```python
from build123d import *

# Parameters (mm, degrees)
SKETCH2_W               = 101.6
SKETCH2_H               = 25.4
BOSS_EXTRUDE1_DEPTH     = 6.35
SKETCH3_R               = 6.35
CUT_EXTRUDE1_DEPTH      = 3.81
CUT_EXTRUDE2_DEPTH      = 53.74706153
CUT_EXTRUDE2_DEPTH_BACK = 6.35
CUT_EXTRUDE3_DEPTH      = 53.74706153
CUT_EXTRUDE3_DEPTH_BACK = 6.35


with BuildPart() as part:
    # Sketch2 → Boss-Extrude1 (new body)
    with BuildSketch(Plane(origin=(0, 0, 0), x_dir=(1, 0, 0), z_dir=(0, 1, 0))):
        Rectangle(SKETCH2_W, SKETCH2_H)
    extrude(amount=BOSS_EXTRUDE1_DEPTH)

    # Sketch3 → Cut-Extrude1 (cut)
    with BuildSketch(Plane.XZ):
        with Locations(Location((-38.1, 0, 0), (0, 0, 270))):
            Circle(SKETCH3_R)
    extrude(amount=-CUT_EXTRUDE1_DEPTH, mode=Mode.SUBTRACT)

    # Sketch4 → Cut-Extrude2 (cut, two sides: drawn at the far end of the back side and taken through both)
    with BuildSketch(Plane(origin=(0, 6.35, 0), x_dir=(1, 0, 0), z_dir=(0, 1, 0)).offset(-CUT_EXTRUDE2_DEPTH_BACK)):
        Polygon((267.54102157, 6.35), (50.8, 6.35), (-25.4, 6.35), (-25.4, 0), (-25.4, -12.7), (-25.4, -229.44102157), (246.403770405, -567.12340506), (539.344791976, -331.332383489), align=None)
    extrude(amount=CUT_EXTRUDE2_DEPTH + CUT_EXTRUDE2_DEPTH_BACK, mode=Mode.SUBTRACT)

    # Sketch5 → Cut-Extrude3 (cut, two sides: drawn at the far end of the back side and taken through both)
    with BuildSketch(Plane(origin=(0, 6.35, 0), x_dir=(1, 0, 0), z_dir=(0, 1, 0)).offset(-CUT_EXTRUDE3_DEPTH_BACK)):
        with BuildLine():
            Line((156.775019491, -16.637334418), (-38.1, -12.7))
            ThreePointArc((-38.1, -12.7), (-50.545995938, 0), (-38.1, 12.7))
            Line((-38.1, 12.7), (156.775019491, 16.637334418))
            Line((156.775019491, 16.637334418), (-233.054562885, 16.637334418))
            Line((-233.054562885, 16.637334418), (-233.054562885, -16.637334418))
            Line((-233.054562885, -16.637334418), (156.775019491, -16.637334418))
        make_face()
    extrude(amount=CUT_EXTRUDE3_DEPTH + CUT_EXTRUDE3_DEPTH_BACK, mode=Mode.SUBTRACT)


solid = part.part
```
Geometry check sheet. Reference: the model listing, model coordinates, mm. A direction names the side the tool comes from. Round coordinates to 2 decimals unless told otherwise and drop trailing zeros. Loops run counter-clockwise (first coordinate to the right, second up) from the corner with the lowest first, then second, coordinate; pieces in that order, holes last. Notation, with made-up numbers: (15.5, 89) - (63.5, 89) arc R25 cw to (63.5, 109) - close; hole circle Ø2 at (1, 35). An arc over 180 degrees is marked (long way). Write item = value, one per line. Start each with the question number.
1. Section check B-B on z = 0. Enter the section's corners in (x, y).
2. Mould release check, pull along Z, two halves, no side actions. Record for faces 4 (the face through (-36.193, 1.878, -6.057)), 5 (the face through (-11, 0, -8)), 6 (the face through (6, 3, -12.7)), 7 (the face through (13, 3, -6.35)): released by +Z, released by -Z, zero draft, split by the parting line, or undercut.
3. Section check C-C on x = 17. Enter the section's corners in (y, z), then the cut area to 3 significant figures.
4. Depth check by flat-ended pin: pin 1 (6.5 mm diameter, centred on x = -41, z = 0.5, fed in from -Y); pin 2 (3 mm diameter, centred on x = 29, y = 1.5, fed in from +Z); pin 3 (10 mm diameter, centred on x = -7, z = -5, fed in from -Y). Enter the tip coordinate at first touch or a pass-through.
5. Set-up check for faces 1 (the face through (-38, 3.81, 0)), 2 (the face through (-32, 3, 12.7)), 3 (the face through (-25.4, 3, 3)): record each of +Z, -Z, +X, -X, +Y, -Y from which the full face is reachable in a straight line by a thin tool's end or side.
6. Thickness scan on line 1 (X direction, y = 2.1, z = 0); line 2 (Z direction, x = 24, y = 1.5); line 3 (Y direction, x = -34.5, z = -5). Record the ranges inside material, lowest first.
7. Section check D-D on z = -4.25. Enter the section's corners in (x, y), then the cut area to 3 significant figures.
Working result:
q1.outline = (-50.55, 0) - (-44.45, 0) - (-44.45, 3.81) - (-31.75, 3.81) - (-31.75, 0) - (-25.4, 0) - (-25.4, 6.35) - (-50.55, 6.35) - close
q2.face_4 = undercut
q2.face_5 = zero draft
q2.face_6 = released by -Z
q2.face_7 = released by +Z
q3.outline = (0, -12.7) - (6.35, -12.7) - (6.35, -6.35) - (0, -6.35) - close
q3.area = 40.3 mm^2
q4.pin_1 = 3.81
q4.pin_2 = -6.35
q4.pin_3 = 0
q5.face_1 = -Y
q5.face_2 = +Z, +X, -X, +Y, -Y
q5.face_3 = +Z, +X, +Y, -Y
q6.line_1 = -50.55 to -44.45, -31.75 to -25.4
q6.line_2 = -12.7 to -6.35
q6.line_3 = 3.81 to 6.35
q7.outline = (-49.81, 0) - (-42.82, 0) - (-42.82, 3.81) - (-33.38, 3.81) - (-33.38, 0) - (-25.4, 0) - (-25.4, 6.35) - (-49.81, 6.35) - close
q7.area = 119 mm^2
